Verification items for this drawing (mm, ordinates from the low corner). A direction names the side the tool comes from. Round coordinates to 2 decimals unless told otherwise and drop trailing zeros. Order: outer loops, then holes, each group sorted by start corner. A loop starts at its lowest first (then second) coordinate and runs counter-clockwise, first axis right, second up. Notation, with made-up numbers: (-22.5, -15) -> (-2.5, -15) arc R11 cw to (-2.5, -11) -> close; hole circle Ø10 at (-26, 47.5). An arc over 180 degrees is marked (long way). Answer in a Markdown table with one row per item.
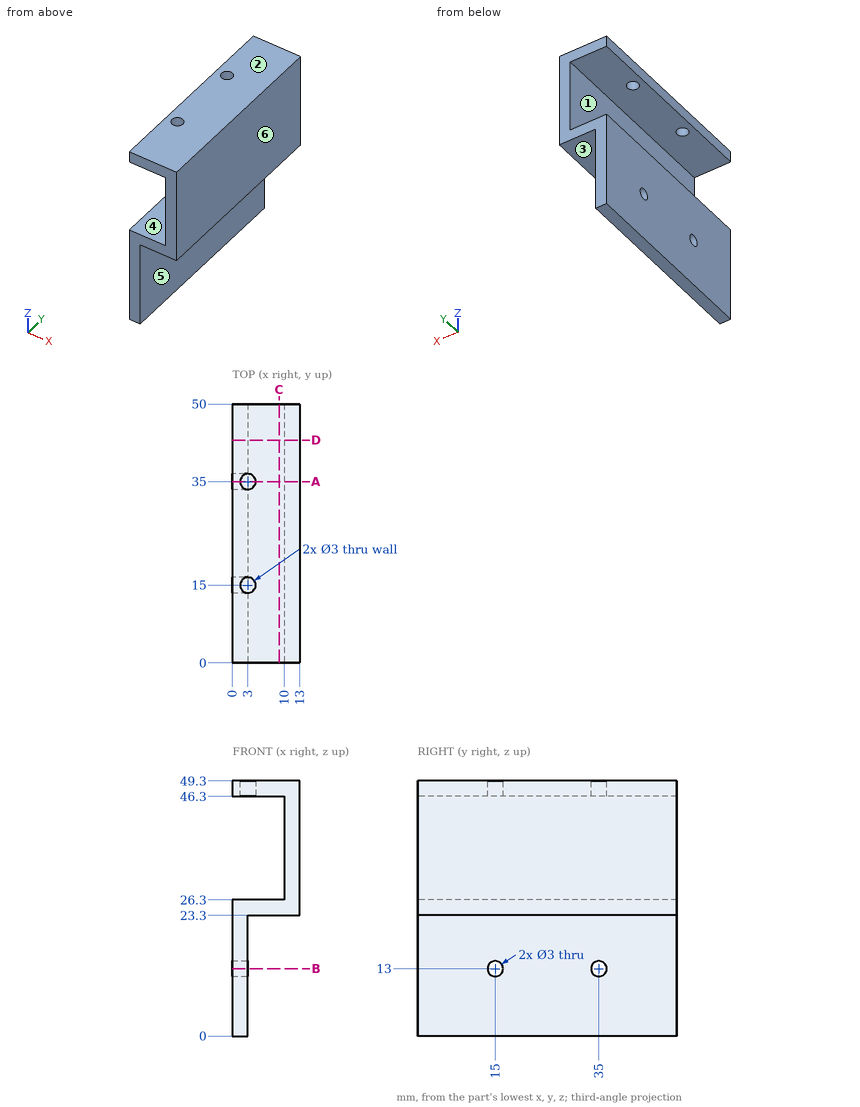
Item 1: Cross-section at A-A (y = 35). Record the boundary of the cut face in (x, z), and give its area (3 significant figures).
Result sheet:
| item | result |
|---|---|
| outline | (0, 0) -> (3, 0) -> (3, 11.5) -> (0, 11.5) -> close; (0, 14.5) -> (3, 14.5) -> (3, 23.3) -> (13, 23.3) -> (13, 49.3) -> (4.5, 49.3) -> (4.5, 46.3) -> (10, 46.3) -> (10, 26.3) -> (0, 26.3) -> close; (0, 46.3) -> (1.5, 46.3) -> (1.5, 49.3) -> (0, 49.3) -> close |
| area | 190 mm^2 |
Item 2: Depth check by flat-ended pin: P1, Ø18.5, axis at y = 21.5, z = 9.5, coming from the +X side; P2, Ø1.5, axis at x = 8, y = 15, coming from the -Z side; P3, Ø6, axis at y = 8, z = 31.5, coming from the -X side. Enter the tip coordinate at first touch or a pass-through.
Result sheet:
| item | result |
|---|---|
| P1 | stops at x = 3 |
| P2 | stops at z = 23.3 |
| P3 | stops at x = 10 |
Item 3: Cross-section at D-D (y = 43). Record the boundary of the cut face in (x, z).
Result sheet:
| item | result |
|---|---|
| outline | (0, 0) -> (3, 0) -> (3, 23.3) -> (13, 23.3) -> (13, 49.3) -> (0, 49.3) -> (0, 46.3) -> (10, 46.3) -> (10, 26.3) -> (0, 26.3) -> close |
Item 4: Mould release check, pull along Z, two halves, no side actions. Record for the marked faces 1, 2 and 3: pulls with the +Z half, pulls with the -Z half, needs draft (parallel to the pull), parting line crosses it, or undercut.
Result sheet:
| item | result |
|---|---|
| face 1 | undercut |
| face 2 | pulls with the +Z half |
| face 3 | pulls with the -Z half |
Item 5: Scan lines: line 1 (Z direction, x = 1.05, y = 35); line 2 (Y direction, x = 3, z = 48.3); line 3 (Z direction, x = 1.5, y = 30). Record each from-to range of solid material in increasing order. Write a range as [from, to].
Result sheet:
| item | result |
|---|---|
| line 1 | z = [0, 11.5], [14.5, 26.3], [46.3, 49.3] |
| line 2 | y = [0, 13.5], [16.5, 33.5], [36.5, 50] |
| line 3 | z = [0, 26.3], [46.3, 49.3] |
Item 6: Cross-section at C-C (x = 9). Record the boundary of the cut face in (y, z), and give its area (3 significant figures).
Result sheet:
| item | result |
|---|---|
| outline | (0, 23.3) -> (50, 23.3) -> (50, 26.3) -> (0, 26.3) -> close; (0, 46.3) -> (50, 46.3) -> (50, 49.3) -> (0, 49.3) -> close |
| area | 300 mm^2 |
Item 7: Set-up check for the marked faces 4, 5 and 6: record each of +Z, -Z, +X, -X, +Y, -Y from which the full face is reachable in a straight line by a thin tool's end or side.
Result sheet:
| item | result |
|---|---|
| face 4 | -X, +Y, -Y |
| face 5 | -Z, +X, +Y, -Y |
| face 6 | +Z, -Z, +X, +Y, -Y |
Item 8: Cross-section at B-B (z = 13). Record the boundary of the cut face in (x, y).
Result sheet:
| item | result |
|---|---|
| outline | (0, 0) -> (3, 0) -> (3, 13.5) -> (0, 13.5) -> close; (0, 16.5) -> (3, 16.5) -> (3, 33.5) -> (0, 33.5) -> close; (0, 36.5) -> (3, 36.5) -> (3, 50) -> (0, 50) -> close |
